Can you work these out from the model? Positions are in its coordinate system, mm. Face numbers are marked on the shaded views. Round coordinates to 2 decimals unless told otherwise and drop trailing zeros. Loops run counter-clockwise (first coordinate to the right, second up) from the corner with the lowest first, then second, coordinate; pieces in that order, holes last. Notation, with made-up numbers: (-6, 79.25) -> (4, 79.25) arc R31 ccw to (4, 114.25) -> close; hole circle Ø10 at (21, 3.25). An arc over 180 degrees is marked (long way). Answer as a JSON object with one key per item and string values.
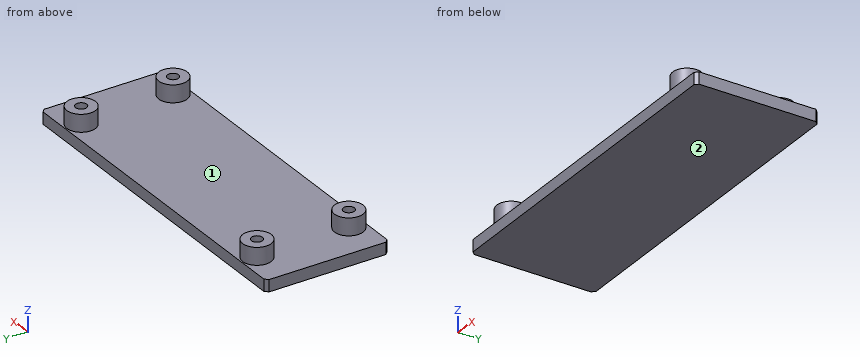
```python
from build123d import *

# Parameters (mm, degrees)
FLAT_BACK_OF_SEPARATELY_PRINTED_SLIDE_IN_DEPTH = 1
PLATE_START                                    = 1
PLATE_RIM_WITH_BLIND_D2_05_PILOT_BOT_2_R       = 1.025
PLATE_RIM_WITH_BLIND_D2_05_PILOT_BOTTOMS_DEPTH = 1.2
RAISED_START                                   = 2.2
RAISED_POWER_BOARD_SUPPORTS_NO_NUT_2_R         = 2.65
RAISED_POWER_BOARD_SUPPORTS_NO_NUT_2_R_2       = 1.025
RAISED_POWER_BOARD_SUPPORTS_NO_NUTS_BE_DEPTH   = 3.2


with BuildPart() as part:
    # Flat back of separately printed slid 2 → Flat back of separately printed slide-in (new body)
    with BuildSketch(Plane.XY):
        Polygon((-31.4, -11.4), (31.4, -11.4), (32, -10.8), (32, 10.8), (31.4, 11.4), (-31.4, 11.4), (-32, 10.8), (-32, -10.8), align=None)
    extrude(amount=FLAT_BACK_OF_SEPARATELY_PRINTED_SLIDE_IN_DEPTH)

    # Plate rim with blind D2.05 pilot bot 2 → Plate rim with blind D2.05 pilot bottoms (add)
    with BuildSketch(Plane.XY.offset(PLATE_START)):
        Polygon((-31.4, -11.4), (31.4, -11.4), (32, -10.8), (32, 10.8), (31.4, 11.4), (-31.4, 11.4), (-32, 10.8), (-32, -10.8), align=None)
        with Locations((-25, -8.5)):
            Circle(PLATE_RIM_WITH_BLIND_D2_05_PILOT_BOT_2_R, mode=Mode.SUBTRACT)
        with Locations((-25, 8.5)):
            Circle(PLATE_RIM_WITH_BLIND_D2_05_PILOT_BOT_2_R, mode=Mode.SUBTRACT)
        with Locations((25, -8.5)):
            Circle(PLATE_RIM_WITH_BLIND_D2_05_PILOT_BOT_2_R, mode=Mode.SUBTRACT)
        with Locations((25, 8.5)):
            Circle(PLATE_RIM_WITH_BLIND_D2_05_PILOT_BOT_2_R, mode=Mode.SUBTRACT)
    extrude(amount=PLATE_RIM_WITH_BLIND_D2_05_PILOT_BOTTOMS_DEPTH)

    # Raised power board supports - no nut 2 → Raised power board supports - no nuts be (add)
    # profile 1 of 4: a face of its own
    with BuildSketch(Plane.XY.offset(RAISED_START)):
        with Locations((-25, -8.5)):
            Circle(RAISED_POWER_BOARD_SUPPORTS_NO_NUT_2_R)
        with Locations((-25, -8.5)):
            Circle(RAISED_POWER_BOARD_SUPPORTS_NO_NUT_2_R_2, mode=Mode.SUBTRACT)
    # profile 2 of 4: a face of its own
    with BuildSketch(Plane.XY.offset(RAISED_START)):
        with Locations((-25, 8.5)):
            Circle(RAISED_POWER_BOARD_SUPPORTS_NO_NUT_2_R)
        with Locations((-25, 8.5)):
            Circle(RAISED_POWER_BOARD_SUPPORTS_NO_NUT_2_R_2, mode=Mode.SUBTRACT)
    # profile 3 of 4: a face of its own
    with BuildSketch(Plane.XY.offset(RAISED_START)):
        with Locations((25, -8.5)):
            Circle(RAISED_POWER_BOARD_SUPPORTS_NO_NUT_2_R)
        with Locations((25, -8.5)):
            Circle(RAISED_POWER_BOARD_SUPPORTS_NO_NUT_2_R_2, mode=Mode.SUBTRACT)
    # profile 4 of 4: a face of its own
    with BuildSketch(Plane.XY.offset(RAISED_START)):
        with Locations((25, 8.5)):
            Circle(RAISED_POWER_BOARD_SUPPORTS_NO_NUT_2_R)
        with Locations((25, 8.5)):
            Circle(RAISED_POWER_BOARD_SUPPORTS_NO_NUT_2_R_2, mode=Mode.SUBTRACT)
    extrude(amount=RAISED_POWER_BOARD_SUPPORTS_NO_NUTS_BE_DEPTH)


solid = part.part
```
Q1. I'm going to push flat-ended pins straight in: pin 1 (3.5 mm diameter, centred on x = 25, y = 8.5, fed in from -Z); pin 2 (3 mm diameter, centred on y = 5, z = 4.5, fed in from +X); pin 3 (0.6 mm diameter, centred on x = -25, y = 8, fed in from +Z). Where does each tip first touch, or does it pass through?
Determined:
{"pin 1": "z = 0", "pin 2": "x = 26.74", "pin 3": "z = 1"}
Q2. I want a section at A-A, the plane y = -8.5. Write out the boundary of the cut face in (x, z) (3 decimals).
Determined:
{"outline": "(-32, 0) -> (32, 0) -> (32, 2.2) -> (27.65, 2.2) -> (27.65, 5.4) -> (26.025, 5.4) -> (26.025, 1) -> (23.975, 1) -> (23.975, 5.4) -> (22.35, 5.4) -> (22.35, 2.2) -> (-22.35, 2.2) -> (-22.35, 5.4) -> (-23.975, 5.4) -> (-23.975, 1) -> (-26.025, 1) -> (-26.025, 5.4) -> (-27.65, 5.4) -> (-27.65, 2.2) -> (-32, 2.2) -> close"}
Q3. I want a section at B-B, the plane x = 25. Write out the boundary of the cut face in (y, z) (3 decimals).
Determined:
{"outline": "(-11.4, 0) -> (11.4, 0) -> (11.4, 2.2) -> (11.15, 2.2) -> (11.15, 5.4) -> (9.525, 5.4) -> (9.525, 1) -> (7.475, 1) -> (7.475, 5.4) -> (5.85, 5.4) -> (5.85, 2.2) -> (-5.85, 2.2) -> (-5.85, 5.4) -> (-7.475, 5.4) -> (-7.475, 1) -> (-9.525, 1) -> (-9.525, 5.4) -> (-11.15, 5.4) -> (-11.15, 2.2) -> (-11.4, 2.2) -> close"}
Q4. I want a section at D-D, the plane x = -5. Write out the boundary of the cut face in (y, z).
Determined:
{"outline": "(-11.4, 0) -> (11.4, 0) -> (11.4, 2.2) -> (-11.4, 2.2) -> close"}
Q5. I want a section at C-C, the plane y = 3.75. Write out the boundary of the cut face in (x, z).
Determined:
{"outline": "(-32, 0) -> (32, 0) -> (32, 2.2) -> (-32, 2.2) -> close"}
Q6. We'd pull the mould along X, two halves only. Please class the marked faces 1 and 2: pulls with the +X half, pulls with the -X half, needs draft (parallel to the pull), parting line crosses it, or undercut.
Determined:
{"face 1": "undercut", "face 2": "needs draft"}
Q7. If I drill on L1, parallel to Y at x = -25, z = 4.4 (3 decimals); L2, parallel to Y at x = 25, z = 1.95 (3 decimals); L3, parallel to Z at x = 2, y = 2.25, over which ranges is the centre line in solid material (lowest first)? Write a range as [from, to].
Determined:
{"L1": "[-11.15, -9.525], [-7.475, -5.85], [5.85, 7.475], [9.525, 11.15]", "L2": "[-11.4, -9.525], [-7.475, 7.475], [9.525, 11.4]", "L3": "[0, 2.2]"}
